Geometry check sheet. Reference: the model listing, model coordinates, mm. Coordinates: 2 decimals unless noted, no trailing zeros. Write each loop counter-clockwise with the first axis right and the second up, starting at its lowest first coordinate (ties: lowest second). Pieces come first, ordered by that corner, then holes. Notation, with made-up numbers: M -33,64.25 L -15,64.25 A29 cw -15,88.25 Z; hole C 37.5,13 d1. An arc over 180 degrees is marked long. Answer as a JSON object with one key per item and string values. Group by question number.
Autodesk Fusion 360 part; units mm, degrees
sketch "草图2" plane through (0, 0, 0) normal (0, 1, 0) x (1, 0, 0)
  line L0 (-9.5492, 29.3893) -> (-9.5492, -29.3893)
  line L1 (-9.5492, -29.3893) -> (25, 18.1636)
  line L2 (25, 18.1636) -> (-30.9017, 0)
  line L3 (-30.9017, 0) -> (25, -18.1636)
  line L4 (25, -18.1636) -> (-9.5492, 29.3893)
  line L5 (-37.5985, -0.9785) -> (29.8427, -22.8914)
  line L6 (30.993, -21.3083) -> (-10.688, 36.0607)
  line L7 (-10.688, -36.0607) -> (30.993, 21.3083)
  line L8 (29.8427, 22.8914) -> (-37.5985, 0.9785)
  line L9 (-12.5492, 35.456) -> (-12.5492, -35.456)
  circle A0 centre (0, 0) radius 40.6112
  circle A1 centre (0, 0) radius 37.6112
  dimension "d2" = 3
extrude "拉伸1" add sketch "草图2" along normal blind 5 contours L0 L4 L6 L8 L9 A1 | L0 L2 L4 L8 | L0 L2 L8 L9 | L2 L4 L6 L8 | L0 L2 L3 L9 | L2 L3 L5 L8 L9 A1 | L1 L2 L4 L6 | L1 L2 L6 L7 L8 A1 | L0 L1 L3 L5 | L0 L3 L5 L9 | L1 L3 L4 L7 | L1 L4 L6 L7 | L0 L1 L5 L7 L9 A1 | L1 L3 L5 L7 | L3 L4 L5 L6 L7 A1 | A0 makes body 1
sketch "草图3" plane through (0, 5, 0) normal (0, 1, 0) x (-1, 0, 0)
  arc A0 (10.688, 36.0607) -> (-29.8427, 22.8914) centre (0, 0) ccw
  line L0 (10.688, 36.0607) -> (-4.7933, 14.7524)
  line L1 (-4.7933, 14.7524) -> (-29.8427, 22.8914)
  line L2 (9.5492, -29.3893) -> (-1.7933, -13.7777)
  line L3 (-1.7933, -13.7777) -> (9.5492, -10.0923)
  line L4 (9.5492, -10.0923) -> (9.5492, -29.3893)
  arc A1 (12.5492, -35.456) -> (37.5985, -0.9785) centre (0, 0) ccw
  line L5 (12.5492, -35.456) -> (12.5492, -9.1175)
  line L6 (12.5492, -9.1175) -> (37.5985, -0.9785)
  line L7 (9.5492, 29.3893) -> (9.5492, 10.0923)
  line L8 (9.5492, 10.0923) -> (-1.7933, 13.7777)
  line L9 (-1.7933, 13.7777) -> (9.5492, 29.3893)
  line L10 (-25, 18.1636) -> (-6.6475, 12.2005)
  line L11 (-6.6475, 12.2005) -> (-13.6575, 2.552)
  line L12 (-13.6575, 2.552) -> (-25, 18.1636)
  line L13 (30.9017, 0) -> (12.5492, -5.9631)
  line L14 (12.5492, -5.9631) -> (12.5492, 5.9631)
  line L15 (12.5492, 5.9631) -> (30.9017, 0)
  arc A2 (37.5985, 0.9785) -> (12.5492, 35.456) centre (0, 0) ccw
  line L16 (37.5985, 0.9785) -> (12.5492, 9.1175)
  line L17 (12.5492, 9.1175) -> (12.5492, 35.456)
  line L18 (-25, -18.1636) -> (-13.6575, -2.552)
  line L19 (-13.6575, -2.552) -> (-6.6475, -12.2005)
  line L20 (-6.6475, -12.2005) -> (-25, -18.1636)
  line L21 (-30.993, 21.3083) -> (-15.5116, 0)
  line L22 (-15.5116, 0) -> (-30.993, -21.3083)
  arc A3 (-30.993, 21.3083) -> (-30.993, -21.3083) centre (0, 0) ccw
  arc A4 (-29.8427, -22.8914) -> (10.688, -36.0607) centre (0, 0) ccw
  line L23 (-29.8427, -22.8914) -> (-4.7933, -14.7524)
  line L24 (-4.7933, -14.7524) -> (10.688, -36.0607)
  line L25 (-11.8034, 0) -> (-3.6475, 11.2257)
  line L26 (-3.6475, 11.2257) -> (9.5492, 6.9379)
  line L27 (9.5492, 6.9379) -> (9.5492, -6.9379)
  line L28 (9.5492, -6.9379) -> (-3.6475, -11.2257)
  line L29 (-3.6475, -11.2257) -> (-11.8034, 0)
  circle A5 centre (0, 0) radius 40.6112
  circle A6 centre (-70, 30) radius 2.5
  circle A7 centre (-70, 30) radius 4
extrude "拉伸2" add sketch "草图3" along normal blind 5 separate body contours A7 makes body 2
move_body "移动1" bodies 2 to x (1, 0, 0) y (0, 1, 0) z (0, 0, 1) at (-85, 0, -75)
move_body "移动2" bodies 2 to x (1, 0, 0) y (0, 1, 0) z (0, 0, 1) at (0, -5, 0)
move_body "移动3" bodies 2 to x (1, 0, 0) y (0, 1, 0) z (0, 0, 1) at (1.5742, 0, 3.989)
combine "合并1" operation add target body 1 tool bodies 2
1) Section check C-C (x = 0). Record the cut outline in (y, z), then the cut area to 3 significant figures.
2) Section check A-A (z = -16.5). Record the cut outline in (x, y).
3) Material ranges on probe 1 along Z at (x, y) = (12.5, 0.8); probe 2 along Z at (x, y) = (-34, 1.8); probe 3 along Z at (x, y) = (-21, 1.2), recorded low to high. Write a range as [from, to].
4) Go/stop test with flat-tipped pins: pin 1 Ø1 at (x, y) = (-30, 3) entering from -Z; pin 2 Ø2.5 at (y, z) = (2, -20) entering from -X; pin 3 Ø2.5 at (y, z) = (2, 26) entering from -X. Record where each tip stops, or that it passes through.
5) Section check D-D (z = -26). Record the cut outline in (x, y), then the cut area to 3 significant figures.
6) Section check B-B (x = 35). Record the cut outline in (y, z), then the cut area to 3 significant figures.
Entries:
{
 "1": {"outline": "M 0,-40.61 L 5,-40.61 L 5,-37.61 L 0,-37.61 Z; M 0,-21.35 L 5,-21.35 L 5,-16.25 L 0,-16.25 Z; M 0,-13.19 L 5,-13.19 L 5,-10.04 L 0,-10.04 Z; M 0,10.04 L 5,10.04 L 5,13.19 L 0,13.19 Z; M 0,16.25 L 5,16.25 L 5,21.35 L 0,21.35 Z; M 0,37.61 L 5,37.61 L 5,40.61 L 0,40.61 Z", "area": "113 mm^2"},
 "2": {"outline": "M -37.11,0 L -33.8,0 L -33.8,5 L -37.11,5 Z; M -12.55,0 L -9.55,0 L -9.55,5 L -12.55,5 Z; M -0.18,0 L 3.52,0 L 3.52,5 L -0.18,5 Z; M 10.17,0 L 19.88,0 L 19.88,5 L 10.17,5 Z; M 23.79,0 L 27.5,0 L 27.5,5 L 23.79,5 Z; M 33.8,0 L 37.11,0 L 37.11,5 L 33.8,5 Z"},
 "3": {"probe 1": "[-38.64, -35.47], [-17.26, -14.1], [-4.15, 4.15], [14.1, 17.26], [35.47, 38.64]", "probe 2": "[-22.21, -16.08], [-2.15, 2.15], [16.08, 22.21]", "probe 3": "[-34.76, -31.2], [-6.37, -3.22], [3.22, 6.37], [31.2, 34.76]"},
 "4": {"pin 1": "z = -27.91", "pin 2": "x = -36.02", "pin 3": "x = -32.2"},
 "5": {"outline": "M -31.2,0 L -27.18,0 L -27.18,5 L -31.2,5 Z; M -12.55,0 L -9.55,0 L -9.55,5 L -12.55,5 Z; M -7.09,0 L -3.38,0 L -3.38,5 L -7.09,5 Z; M 27.18,0 L 31.2,0 L 31.2,5 L 27.18,5 Z", "area": "73.7 mm^2"},
 "6": {"outline": "M 0,-20.6 L 5,-20.6 L 5,-13.77 L 0,-13.77 Z; M 0,13.77 L 5,13.77 L 5,20.6 L 0,20.6 Z", "area": "68.3 mm^2"}
}
